```python
from build123d import *

# Parameters (mm, degrees)
T_LE_DE_BASE_PLI_E1_DEPTH              = 3
TENON_START                            = 14.9
TENON_ET_MORTAISE_RAINURE1_OUTLINE_W   = 3.1
TENON_ET_MORTAISE_RAINURE1_OUTLINE_H   = 3
TENON_ET_MORTAISE_RAINURE1_DEPTH       = 10.2
TENON_ET_MORTAISE_RAINURE1_2_OUTLINE_W = 3.1
TENON_ET_MORTAISE_RAINURE1_2_OUTLINE_H = 3
TENON_ET_MORTAISE_RAINURE1_2_DEPTH     = 10.1
TENON_START_2                          = 29.9
TENON_ET_MORTAISE_RAINURE1_3_OUTLINE_W = 3.1
TENON_ET_MORTAISE_RAINURE1_3_OUTLINE_H = 3
TENON_ET_MORTAISE_RAINURE1_3_DEPTH     = 10.1


# Read off the part's stored shape, not the designer's step: Tenon et mortaise-Rainure1
# Sheet-metal steps are written as plain solids
with BuildPart() as part:
    # Esquisse1 → Tôle de base pliée1 (new body)
    with BuildSketch(Plane.XY):
        Polygon((25, 0), (115, 0), (115, 40), (0, 40), align=None)
    extrude(amount=T_LE_DE_BASE_PLI_E1_DEPTH)

    # Tenon et mortaise-Rainure1 outline → Tenon et mortaise-Rainure1 (cut)
    with BuildSketch(Plane(origin=(0, 0, 0), x_dir=(1, 0, 0), z_dir=(0, 1, 0)).offset(TENON_START)):
        with Locations((113.45, -1.5)):
            Rectangle(TENON_ET_MORTAISE_RAINURE1_OUTLINE_W, TENON_ET_MORTAISE_RAINURE1_OUTLINE_H)
    extrude(amount=TENON_ET_MORTAISE_RAINURE1_DEPTH, mode=Mode.SUBTRACT)

    # Tenon et mortaise-Rainure1 2 outline → Tenon et mortaise-Rainure1 2 (cut)
    with BuildSketch(Plane(origin=(0, 0, 0), x_dir=(1, 0, 0), z_dir=(0, 1, 0))):
        with Locations((113.45, -1.5)):
            Rectangle(TENON_ET_MORTAISE_RAINURE1_2_OUTLINE_W, TENON_ET_MORTAISE_RAINURE1_2_OUTLINE_H)
    extrude(amount=TENON_ET_MORTAISE_RAINURE1_2_DEPTH, mode=Mode.SUBTRACT)

    # Tenon et mortaise-Rainure1 3 outline → Tenon et mortaise-Rainure1 3 (cut)
    with BuildSketch(Plane(origin=(0, 0, 0), x_dir=(1, 0, 0), z_dir=(0, 1, 0)).offset(TENON_START_2)):
        with Locations((113.45, -1.5)):
            Rectangle(TENON_ET_MORTAISE_RAINURE1_3_OUTLINE_W, TENON_ET_MORTAISE_RAINURE1_3_OUTLINE_H)
    extrude(amount=TENON_ET_MORTAISE_RAINURE1_3_DEPTH, mode=Mode.SUBTRACT)


solid = part.part
```
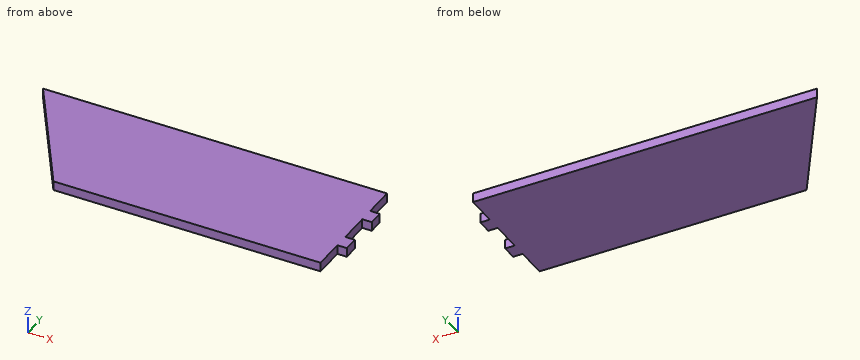
Geometry: final body of the model. Coordinates: model frame, mm. Coordinates: 2 decimals unless noted, no trailing zeros. Write each loop counter-clockwise with the first axis right and the second up, starting at its lowest first coordinate (ties: lowest second). Pieces come first, ordered by that corner, then holes. Notation, with made-up numbers: M 69.5,45 L 109.5,45 A19 ccw 109.5,58 Z; hole C 50,4.25 d3. An arc over 180 degrees is marked long. Use CSV: the item, a comma, the result in double quotes. Start each with the question number.
1. Cut plane A-A on z = 0.85. Return the cut outline in (x, y).
2. Cut plane C-C on y = 37. Return the cut outline in (x, z) (3 decimals).
3. Ray query, probe 1 along X at (y, z) = (9.5, 0.3); probe 2 along X at (y, z) = (3.5, 1.45); probe 3 along Y at (x, z) = (17.5, 2.35). Return the intervals inside material, ascending.
4. First-contact query: P1, Ø1, axis at y = 4, z = 2.5, coming from the -X side; P2, Ø0.9, axis at x = 114, z = 1, coming from the +Y side; P3, Ø1.5, axis at y = 5, z = 1, coming from the +X side. Flat tips, straight axial feed; report the tip coordinate or a pass-through.
5. Cut plane B-B on y = 12. Return the cut outline in (x, z).
Entries:
1,outline,"M 0,40 L 25,0 L 111.9,0 L 111.9,10.1 L 115,10.1 L 115,14.9 L 111.9,14.9 L 111.9,25.1 L 115,25.1 L 115,29.9 L 111.9,29.9 L 111.9,40 Z"
2,outline,"M 1.875,0 L 111.9,0 L 111.9,3 L 1.875,3 Z"
3,probe 1,"19.06 to 111.9"
3,probe 2,"22.81 to 111.9"
3,probe 3,"12 to 40"
4,P1,"x = 22.19"
4,P2,"y = 29.9"
4,P3,"x = 111.9"
5,outline,"M 17.5,0 L 115,0 L 115,3 L 17.5,3 Z"
